Autodesk Inventor part; units mm, degrees
ref_plane "YZ Plane" through (0, 0, 0) normal (1, 0, 0) x (0, 1, 0)
ref_plane "XZ Plane" through (0, 0, 0) normal (0, 1, 0) x (-1, 0, 0)
ref_plane "XY Plane" through (0, 0, 0) normal (0, 0, 1) x (1, 0, 0)
sketch "Sketch1" plane through (0, 0, 0) normal (0, 1, 0) x (-1, 0, 0)
  line L0 (19.5, -173) -> (0, -173) construction
  line L1 (0, -173) -> (-19.5, -173) construction
  line L2 (61, -173) -> (61, 35)
  line L3 (0, 0) -> (0, -173) construction
  line L4 (0, -188) -> (30, -188)
  line L5 (61, -173) -> (30, -188)
  line L6 (61, 35) -> (0, 41)
  line L7 (-61, -173) -> (-61, 35)
  line L8 (0, -188) -> (-30, -188)
  line L9 (-61, -173) -> (-30, -188)
  line L10 (-61, 35) -> (0, 41)
  point P0 (0, -118)
  point P1 (0, -158)
  dimension "d0" = 118
  dimension "d1" = 40
  dimension "d2" = 19.5
  dimension "d3" = 15
  dimension "d4" = 61
  dimension "d6" = 15
  dimension "d7" = 35
  dimension "d8" = 41
  dimension "d11" = 30
extrude "uitlijn plaatje" add sketch "Sketch1" along normal blind 10
hole "Hole1" at (-19.5, 0, -173) at (19.5, 0, -173) at (0, 0, 0) at (0, 0, -118) at (0, 0, -158) direction (0, 1, 0) diameter 3.4 end through all
sketch "batterij uitsnijding" plane through (0, 10, 0) normal (0, 1, 0) x (1, 0, 0)
  line L0 (-61, -35) -> (0, -41)
  line L1 (-16, -39.4262) -> (-16, 112)
  line L2 (-16, 112) -> (-61, 112)
  line L3 (-61, 173) -> (-61, -35)
  point P0 (0, 0)
  dimension "d21" = 45
  dimension "d22" = 112
extrude "Extrusion2" cut sketch "batterij uitsnijding" against normal blind 10
sketch "Sketch3" plane through (0, 10, 0) normal (0, 1, 0) x (1, 0, 0)
  circle A0 centre (25.75, 14.75) radius 5
  point P0 (0, 0)
  dimension "d26" = 14.75
  dimension "d27" = 25.75
  dimension "d28" = 10
extrude "Extrusion3" cut sketch "Sketch3" against normal blind 10
sketch "Sketch4" plane through (0, 10, 0) normal (0, 1, 0) x (1, 0, 0)
  line L0 (56.6557, 151.7192) -> (-9.4519, 151.7192)
  line L1 (-9.4519, 151.7192) -> (-9.4519, 66.7192)
  line L2 (-9.4519, 66.7192) -> (56.6557, 66.7192)
  line L3 (56.6557, 66.7192) -> (56.6557, 151.7192)
  point P0 (0, 0)
  point P1 (0, -30.4368)
  point P2 (0, 9.5632)
  point P3 (45, -30.4368)
  point P4 (45, 9.5632)
  point P5 (51.8228, 48.7167)
  point P6 (51.8228, 29.7167)
  point P7 (-3.1772, 48.7167)
  point P8 (-3.1772, 29.7167)
  point P9 (5.7892, 70.2192)
  point P10 (54.7892, 70.2192)
  point P11 (54.7892, 128.2192)
  point P12 (5.7892, 128.2192)
  dimension "d31" = 40
  dimension "d32" = 45
  dimension "d33" = 19
  dimension "d34" = 55
  dimension "d35" = 58
  dimension "d36" = 49
  dimension "d37" = 55
  dimension "d38" = 19
  dimension "d39" = 85
  dimension "d40" = 3.5
hole "Hole2" at (0, 10, 30.4368) at (0, 10, -9.5632) at (45, 10, 30.4368) at (45, 10, -9.5632) at (51.8228, 10, -48.7167) at (51.8228, 10, -29.7167) at (-3.1772, 10, -48.7167) at (-3.1772, 10, -29.7167) at (5.7892, 10, -70.2192) at (54.7892, 10, -70.2192) at (54.7892, 10, -128.2192) at (5.7892, 10, -128.2192) direction (0, -1, 0) diameter 2.2 end through all
sketch "Sketch5" plane through (0, 10, 0) normal (0, 1, 0) x (1, 0, 0)
  line L0 (0, -41) -> (61, -35)
  line L1 (51, -35.9836) -> (51, -23.9836)
  line L2 (51, -23.9836) -> (39, -23.9836)
  line L3 (39, -23.9836) -> (39, 1.0164)
  line L4 (39, 1.0164) -> (54.3101, 1.0164)
  line L5 (54.3101, 1.0164) -> (61, 1.0164)
  line L6 (61, -35) -> (61, 173)
  point P0 (0, 0)
  dimension "d48" = 25
  dimension "d49" = 12
  dimension "d50" = 10
  dimension "d51" = 12
extrude "Extrusion4" cut sketch "Sketch5" against normal blind 10
properties part number "montageplaatje"
The model under review builds one solid part; all positions refer to its coordinate system, in mm. A direction names the side the tool comes from. Round coordinates to 2 decimals unless told otherwise and drop trailing zeros. Write each loop counter-clockwise with the first axis right and the second up, starting at its lowest first coordinate (ties: lowest second). Pieces come first, ordered by that corner, then holes.
(1) We need section B-B on z = -14.75. Give the boundary of the cut face in (x, y), and give its area (3 significant figures).
(2) We need section D-D on z = -61. Give the boundary of the cut face in (x, y).
(3) We need section A-A on x = 25.75. Give the boundary of the cut face in (y, z), and give its area (3 significant figures).
(4) Wall thickness on L1, parallel to X at y = 3.5, z = 30.5; L2, parallel to Z at x = 0, y = 6.25; L3, parallel to X at y = 6.5, z = -173: over which ranges is each line inside the solid? List them lowest first.
(5) Mouldability with a two-part tool opening along Z and no side actions: class faces 4 (the flat face through (45.717, 4.93, -180.395)), 5 (the flat face through (45, 5, 23.984)), 6 (the flat face through (-8.112, 4.93, 40.202)) as +Z half, -Z half, draft (parallel to the pull), parting line (faces both ways), or undercut.
(6) Machinability: for faces 1 (the flat face through (51, 5, 30)), 2 (the flat face through (-38, 5, -112)), 3 (the flat face through (50, 5, -1.016)), which of the approach directions +Z, -Z, +X, -X, +Y, -Y give a long, thin tool a straight path to every point of the face, cutting with its end or side? Answer none if there is none.
(7) Insertion check: pin 1 (1.8 mm diameter, centred on x = 54.79, z = -70.22, fed in from -Y); pin 2 (5 mm diameter, centred on y = 8.5, z = 5, fed in from -X); pin 3 (2 mm diameter, centred on x = 33.5, y = 1.5, fed in from +Z); pin 4 (3 mm diameter, centred on x = 46, y = 7, fed in from -Z). Each pin has a flat end and moves straight along its axis. Give the tip position at first contact, or say it passes through.
(8) We need section C-C on y = 5.75. Give the number of separate pieces and of enclosed holes in the cut face, and give its area (3 significant figures).
Findings below:
1. outline: (-16, 0) - (20.75, 0) - (20.75, 10) - (-16, 10) - close; (30.75, 0) - (61, 0) - (61, 10) - (30.75, 10) - close
1. area: 670 mm2
2. outline: (-16, 0) - (61, 0) - (61, 10) - (-16, 10) - close
3. outline: (0, -188) - (10, -188) - (10, -19.75) - (0, -19.75) - close; (0, -9.75) - (10, -9.75) - (10, 38.47) - (0, 38.47) - close
3. area: 2,160 mm2
4. L1: x = -16 to -1.1, 1.1 to 43.9, 46.1 to 51
4. L2: z = -188 to -159.7, -156.3 to -119.7, -116.3 to -10.66, -8.46 to -1.7, 1.7 to 29.34, 31.54 to 41
4. L3: x = -61 to -21.2, -17.8 to 17.8, 21.2 to 61
5. face 4: -Z half
5. face 5: undercut
5. face 6: +Z half
6. face 1: +Z, +X, +Y, -Y
6. face 2: +Z, -X, +Y, -Y
6. face 3: +X, +Y, -Y
7. pin 1: passes through
7. pin 2: stops at x = -16
7. pin 3: stops at z = 37.8
7. pin 4: stops at z = -180.98
8. separate pieces: 1
8. enclosed holes: 18
8. area: 19,600 mm2
